Build history of the part. All positions in model axes, mm. A direction names the side the tool comes from. Round coordinates to 2 decimals unless told otherwise and drop trailing zeros. Write each loop counter-clockwise with the first axis right and the second up, starting at its lowest first coordinate (ties: lowest second). Pieces come first, ordered by that corner, then holes.
1) Saw through at C-C (y = 4.75). State how many separate pieces and enclosed holes the cut face has, plus the area to 3 significant figures.
2) Flat gauge pins, fed straight in: pin 1 (2.5 mm diameter, centred on x = 37.07, z = 22.93, fed in from -Y); pin 2 (5 mm diameter, centred on x = -25, z = 24, fed in from -Y); pin 3 (3 mm diameter, centred on y = 8.5, z = -50, fed in from -X); pin 4 (11 mm diameter, centred on x = -4.5, z = -49, fed in from +Y). Where does each tip first touch, or does it go through?
3) Saw through at D-D (x = 50). Write the cut outline in (y, z), plus the area to 3 significant figures.
4) Pull direction X, two halves, no side cores. Call faces 3 (the flat face through (0, 2.5, 50)), 4 (the cylindrical face through (-35.926, 5.07, 36.797)), 5 (the cylindrical face through (75, 5, 0)), 6 (the cylindrical face through (-38.846, 6.302, -1.465)): +X half, -X half, draft (parallel to the pull), parting line (faces both ways), or undercut.
5) Saw through at B-B (x = -30). Write the cut outline in (y, z), plus the area to 3 significant figures.
6) Which spindle directions (+Z, -Z, +X, -X, +Y, -Y) get a long thin tool onto all of the face, cutting with end or side? Do faces 1 (the flat face through (18, 10, -18)), 2 (the flat face through (0, 2.5, -50)). Say none if no direction does.
7) Wall check: probe 1 along X at (y, z) = (6.25, 0); probe 2 along X at (y, z) = (6.5, 7.5); probe 3 along X at (y, z) = (3.5, 30). Give the ranges that are in metal, low to high.
8) Saw through at A-A (z = 0). Write the cut outline in (x, y), plus the area to 4 significant figures.
from build123d import *

# Parameters (mm, degrees)
SKETCH1_R           = 75
BOSS_EXTRUDE1_DEPTH = 10
SKETCH4_R           = 90
CUT_EXTRUDE2_DEPTH  = 10
SKETCH5_R           = 2.5
SKETCH5_R_2         = 25
SKETCH5_R_3         = 1.5
CUT_EXTRUDE3_DEPTH  = 10
SKETCH6_R           = 1.5
CUT_EXTRUDE4_DEPTH  = 10
SKETCH8_R           = 11.25
CUT_EXTRUDE5_DEPTH  = 7.5


with BuildPart() as part:
    # Sketch1 → Boss-Extrude1 (new body)
    with BuildSketch(Plane(origin=(0, 0, 0), x_dir=(1, 0, 0), z_dir=(0, 1, 0))):
        with Locations(Location((0, 0, 0), (0, 0, 270))):
            Circle(SKETCH1_R)
    extrude(amount=BOSS_EXTRUDE1_DEPTH)

    # Sketch4 → Cut-Extrude2 (cut)
    with BuildSketch(Plane(origin=(0, 10, 0), x_dir=(1, 0, 0), z_dir=(0, 1, 0))):
        with Locations((-100, 100)):
            Circle(SKETCH4_R)
        with Locations((100, 100)):
            Circle(SKETCH4_R)
        with Locations((100, -100)):
            Circle(SKETCH4_R)
        with Locations((-100, -100)):
            Circle(SKETCH4_R)
    extrude(amount=-CUT_EXTRUDE2_DEPTH, mode=Mode.SUBTRACT)

    # Sketch5 → Cut-Extrude3 (cut)
    with BuildSketch(Plane(origin=(0, 10, 0), x_dir=(1, 0, 0), z_dir=(0, 1, 0))):
        with Locations(Location((-30, 30, 0), (0, 0, 270))):
            Circle(SKETCH5_R)
        with Locations(Location((30, 30, 0), (0, 0, 270))):
            Circle(SKETCH5_R)
        with Locations(Location((30, -30, 0), (0, 0, 270))):
            Circle(SKETCH5_R)
        with Locations(Location((-30, -30, 0), (0, 0, 270))):
            Circle(SKETCH5_R)
        with Locations(Location((0, 0, 0), (0, 0, 270))):
            Circle(SKETCH5_R_2)
        with Locations(Location((-37.071067812, -22.928932188, 0), (0, 0, 270))):
            Circle(SKETCH5_R_3)
        with Locations(Location((-22.928932188, -37.071067812, 0), (0, 0, 270))):
            Circle(SKETCH5_R_3)
        with Locations(Location((22.928932188, -37.071067812, 0), (0, 0, 270))):
            Circle(SKETCH5_R_3)
        with Locations(Location((37.071067812, -22.928932188, 0), (0, 0, 270))):
            Circle(SKETCH5_R_3)
        with Locations(Location((37.071067812, 22.928932188, 0), (0, 0, 270))):
            Circle(SKETCH5_R_3)
        with Locations(Location((22.928932188, 37.071067812, 0), (0, 0, 270))):
            Circle(SKETCH5_R_3)
        with Locations(Location((-22.928932188, 37.071067812, 0), (0, 0, 270))):
            Circle(SKETCH5_R_3)
        with Locations(Location((-37.071067812, 22.928932188, 0), (0, 0, 270))):
            Circle(SKETCH5_R_3)
    extrude(amount=-CUT_EXTRUDE3_DEPTH, mode=Mode.SUBTRACT)

    # Sketch6 → Cut-Extrude4 (cut)
    with BuildSketch(Plane(origin=(0, 10, 0), x_dir=(1, 0, 0), z_dir=(0, 1, 0))):
        with Locations(Location((-25, 25, 0), (0, 0, 270))):
            Circle(SKETCH6_R)
        with Locations(Location((25, 25, 0), (0, 0, 270))):
            Circle(SKETCH6_R)
        with Locations(Location((25, -25, 0), (0, 0, 270))):
            Circle(SKETCH6_R)
        with Locations(Location((-25, -25, 0), (0, 0, 270))):
            Circle(SKETCH6_R)
    extrude(amount=-CUT_EXTRUDE4_DEPTH, mode=Mode.SUBTRACT)

    # Sketch8 → Cut-Extrude5 (cut)
    with BuildSketch(Plane(origin=(0, 10, 0), x_dir=(1, 0, 0), z_dir=(0, 1, 0))):
        with Locations(Location((-50, 0, 0), (0, 0, 270))):
            Circle(SKETCH8_R)
        with Locations(Location((0, 50, 0), (0, 0, 270))):
            Circle(SKETCH8_R)
        with Locations(Location((50, 0, 0), (0, 0, 270))):
            Circle(SKETCH8_R)
        with Locations(Location((0, -50, 0), (0, 0, 270))):
            Circle(SKETCH8_R)
    extrude(amount=-CUT_EXTRUDE5_DEPTH, mode=Mode.SUBTRACT)


solid = part.part
Evaluation:
1. separate pieces: 1
1. enclosed holes: 21
1. area: 8,560 mm2
2. pin 1: passes through
2. pin 2: stops at y = 0
2. pin 3: stops at x = -26.19
2. pin 4: stops at y = 2.5
3. outline: (0, -25.17) - (10, -25.17) - (10, -11.25) - (2.5, -11.25) - (2.5, 11.25) - (10, 11.25) - (10, 25.17) - (0, 25.17) - close
3. area: 335 mm2
4. face 3: undercut
4. face 4: -X half
4. face 5: +X half
4. face 6: undercut
5. outline: (0, -43.43) - (10, -43.43) - (10, -32.5) - (0, -32.5) - close; (0, -27.5) - (10, -27.5) - (10, 27.5) - (0, 27.5) - close; (0, 32.5) - (10, 32.5) - (10, 43.43) - (0, 43.43) - close
5. area: 769 mm2
6. face 1: +Z, -Z, +X, -X, +Y
6. face 2: +Y
7. probe 1: x = -75 to -61.25, -38.75 to -25, 25 to 38.75, 61.25 to 75
7. probe 2: x = -74.62 to -58.39, -41.61 to -23.85, 23.85 to 41.61, 58.39 to 74.62
7. probe 3: x = -43.43 to -32.5, -27.5 to 27.5, 32.5 to 43.43
8. outline: (-75, 0) - (-25, 0) - (-25, 10) - (-38.75, 10) - (-38.75, 2.5) - (-61.25, 2.5) - (-61.25, 10) - (-75, 10) - close; (25, 0) - (75, 0) - (75, 10) - (61.25, 10) - (61.25, 2.5) - (38.75, 2.5) - (38.75, 10) - (25, 10) - close
8. area: 662.5 mm2
